Source: CAD feature listing. Evaluate the final solid. Frame: model axes, mm. Give positions to 0.01 mm unless a question says otherwise; leave off trailing zeros. Order: outer loops, then holes, each group sorted by start corner. A loop starts at its lowest first (then second) coordinate and runs counter-clockwise, first axis right, second up. Notation, with made-up numbers: M 5.5,22 L 53.5,22 A20 ccw 53.5,46 Z; hole C 81,-25 d9. An arc over 180 degrees is marked long. Return JSON: item names as keys, results as strings.
from build123d import *

# Parameters (mm, degrees)
BOSS_EXTRUDE1_DEPTH = 6.35
FILLET1_R           = 6.35


with BuildPart() as part:
    # Sketch1 → Boss-Extrude1 (new body)
    with BuildSketch(Plane(origin=(0, 0, 0), x_dir=(1, 0, 0), z_dir=(0, 1, 0))):
        with BuildLine():
            Line((0, 0), (0, 228.6))
            Line((0, 228.6), (-317.5, 228.6))
            Line((-317.5, 228.6), (-317.5, 190.5))
            ThreePointArc((-317.5, 190.5), (-153.625703663, 137.984014872), (-50.8, 0))
            Line((-50.8, 0), (0, 0))
        make_face()
    extrude(amount=BOSS_EXTRUDE1_DEPTH)

    # Fillet1
    fillet1_edges = [part.edges().sort_by_distance(p)[0] for p in [
        (-50.8, 3.175, 0),
        (-317.5, 3.175, -190.5),
        (-317.5, 3.175, -228.6),
        (0, 3.175, -228.6),
        (0, 3.175, 0),
    ]]
    fillet(fillet1_edges, radius=FILLET1_R)


solid = part.part
1. Ray query, probe 1 along Z at (x, y) = (-83.5, 4); probe 2 along Z at (x, y) = (-146, 1.75); probe 3 along X at (y, z) = (5.25, -79). Return the intervals inside material, ascending.
Evaluation:
{"probe 1": "z = -228.6 to -65.83", "probe 2": "z = -228.6 to -132.34", "probe 3": "x = -92.91 to 0"}
2. Section query A-A (y = 3.25). Return loops of the section in (x, z), then the cut area to 3 significant figures.
Evaluation:
{"outline": "M -317.5,-222.25 A6.35 ccw -311.15,-228.6 L -6.35,-228.6 A6.35 ccw 0,-222.25 L 0,-6.35 A6.35 ccw -6.35,0 L -46.3,0 A6.35 ccw -52.28,-4.2 A281.94 cw -311.29,-190.43 A6.35 ccw -317.5,-196.78 Z", "area": "35,400 mm^2"}
3. Section query B-B (x = -160.5). Return loops of the section in (y, z).
Evaluation:
{"outline": "M 0,-228.6 L 6.35,-228.6 L 6.35,-142.74 L 0,-142.74 Z"}
4. First-contact query: pin 1 (1.5 mm diameter, centred on x = -177.5, y = 0.5, fed in from +Z). Flat tip, straight axial feed; report the tip coordinate or a pass-through.
Evaluation:
{"pin 1": "stops at z = -152.85"}
5. Section query C-C (z = -143). Return loops of the section in (x, y).
Evaluation:
{"outline": "M -160.89,0 L 0,0 L 0,6.35 L -160.89,6.35 Z"}
